from build123d import *

# Parameters (mm, degrees)
SKETCH_1_W          = 86
SKETCH_1_H          = 86
EXTRUDE_1_DEPTH     = 1
SKETCH_2_W          = 80
SKETCH_2_H          = 80
CUT_EXTRUDE_1_DEPTH = 61.819404798
SKETCH_3_W          = 86
SKETCH_3_H          = 86
SKETCH_3_W_2        = 82
SKETCH_3_H_2        = 82
EXTRUDE_2_DEPTH     = 5
CHAMFER_1_SIZE      = 1
FILLET_1_R          = 2


with BuildPart() as part:
    # 草图1 → 凸台-拉伸1 (new body)
    with BuildSketch(Plane(origin=(0, 0, 0), x_dir=(1, 0, 0), z_dir=(0, 1, 0))):
        Rectangle(SKETCH_1_W, SKETCH_1_H)
    extrude(amount=EXTRUDE_1_DEPTH)

    # 草图2 → 切除-拉伸1 (cut, through all)
    with BuildSketch(Plane.XZ):
        Rectangle(SKETCH_2_W, SKETCH_2_H)
    extrude(amount=-CUT_EXTRUDE_1_DEPTH, mode=Mode.SUBTRACT)

    # 草图3 → 凸台-拉伸2 (add)
    with BuildSketch(Plane(origin=(0, 1, 0), x_dir=(1, 0, 0), z_dir=(0, 1, 0))):
        Rectangle(SKETCH_3_W, SKETCH_3_H)
        Rectangle(SKETCH_3_W_2, SKETCH_3_H_2, mode=Mode.SUBTRACT)
    extrude(amount=EXTRUDE_2_DEPTH)

    # 倒角1
    chamfer_1_edges = [part.edges().sort_by_distance(p)[0] for p in [
        (0, 0, 43),
        (43, 0, 0),
        (0, 0, -43),
        (-43, 0, 0),
    ]]
    chamfer(chamfer_1_edges, length=CHAMFER_1_SIZE)

    # 圆角1
    fillet_1_edges = [part.edges().sort_by_distance(p)[0] for p in [
        (-43, 3.5, 43),
        (43, 3.5, 43),
        (43, 3.5, -43),
        (-43, 3.5, -43),
    ]]
    fillet(fillet_1_edges, radius=FILLET_1_R)


solid = part.part
The model under review builds one solid part; all positions refer to its coordinate system, in mm. A direction names the side the tool comes from. Give positions to 0.01 mm unless a question says otherwise; leave off trailing zeros. Loops run counter-clockwise (first coordinate to the right, second up) from the corner with the lowest first, then second, coordinate; pieces in that order, holes last. Notation, with made-up numbers: (35, 60.25) -> (41, 60.25) arc R30 ccw to (41, 89.25) -> close; hole circle Ø3 at (-5.75, 75). An arc over 180 degrees is marked (long way). Write each question's results on one line, items separated by ' | '.
1) Take a section at B-B, the plane z = 0.5. Give the boundary of the cut face in (x, y).
Conclusion:
outline: (-43, 1) -> (-42, 0) -> (-40, 0) -> (-40, 1) -> (-41, 1) -> (-41, 6) -> (-43, 6) -> close; (40, 0) -> (42, 0) -> (43, 1) -> (43, 6) -> (41, 6) -> (41, 1) -> (40, 1) -> close
2) Tool access review of faces 1 (the face through (-42.43, 3.17, -42.4)), 2 (the face through (41, 3, 1)): name each direction out of +Z, -Z, +X, -X, +Y, -Y from which nothing blocks a thin tool from reaching the whole face with its end or side.
Conclusion:
face 1: -Z, -X, +Y, -Y | face 2: +Y
3) Insertion check: pin 1 Ø1.1 at (x, y) = (-18.5, 0.5) entering from -Z; pin 2 Ø0.5 at (y, z) = (0.5, 12) entering from +X; pin 3 Ø0.8 at (y, z) = (0.5, 18) entering from -X. Each pin has a flat end and moves straight along its axis. Give the tip position at first contact, or say it passes through.
Conclusion:
pin 1: stops at z = -43 | pin 2: stops at x = 42.75 | pin 3: stops at x = -42.9
4) Take a section at A-A, the plane x = 4. Give the boundary of the cut face in (y, z), plus the area to 3 significant figures.
Conclusion:
outline: (0, -42) -> (1, -43) -> (6, -43) -> (6, -41) -> (1, -41) -> (1, -40) -> (0, -40) -> close; (0, 40) -> (1, 40) -> (1, 41) -> (6, 41) -> (6, 43) -> (1, 43) -> (0, 42) -> close | area: 25.0 mm^2
5) Draft analysis for pull direction Z (two halves, no side actions). For faces 3 (the face through (-1, 3, -43)), 4 (the face through (-3.3, 0, 40.2)), 5 (the face through (-41, 3, 1)), state which applies: pulls with the +Z half, pulls with the -Z half, needs draft (parallel to the pull), parting line crosses it, or undercut.
Conclusion:
face 3: pulls with the -Z half | face 4: needs draft | face 5: undercut
6) For line 1 along Z through (x, y) = (18, 2); line 2 along X through (y, z) = (0.45, 23.5), list the stretches that pass through material, from the lowest coordinate up. Write a range as from..to.
Conclusion:
line 1: z = -43..-41, 41..43 | line 2: x = -42.45..-40, 40..42.45
7) Take a section at C-C, the plane y = 4.15. Give the boundary of the cut face in (x, z).
Conclusion:
outline: (-43, -41) arc R2 ccw to (-41, -43) -> (41, -43) arc R2 ccw to (43, -41) -> (43, 41) arc R2 ccw to (41, 43) -> (-41, 43) arc R2 ccw to (-43, 41) -> close; hole (-41, -41) -> (41, -41) -> (41, 41) -> (-41, 41) -> close
